Autodesk Inventor part; units mm, degrees
ref_plane "Work Plane2" through (46, 0, 0) normal (1, 0, 0) x (0, 1, 0)
ref_plane "XZ Plane" through (0, 0, 0) normal (0, 1, 0) x (-1, 0, 0)
ref_plane "XY Plane" through (0, 0, 0) normal (0, 0, 1) x (1, 0, 0)
sketch "Sketch1" plane through (0, 0, 0) normal (0, 1, 0) x (-1, 0, 0)
  circle A0 centre (0, 0) radius 46
  dimension "d0" = 92
extrude "Extrusion1" add sketch "Sketch1" along normal blind 20
sketch "Sketch2" plane through (0, 20, 0) normal (0, 1, 0) x (1, 0, 0)
  circle A0 centre (0, 0) radius 33
  dimension "d3" = 66
extrude "Extrusion2" cut sketch "Sketch2" against normal blind 14
sketch "Sketch3" plane through (0, 6, 0) normal (0, 1, 0) x (1, 0, 0)
  circle A0 centre (0, 0) radius 2.5
  dimension "d6" = 5
extrude "Extrusion3" cut sketch "Sketch3" against normal blind 6
sketch "Sketch4" plane through (0, 0, 0) normal (0, -1, 0) x (1, 0, 0)
  circle A0 centre (0, 0) radius 12
  dimension "d9" = 24
extrude "Extrusion4" add sketch "Sketch4" along normal blind 10
sketch "Sketch5" plane through (0, 0, 0) normal (0, -1, 0) x (1, 0, 0)
  circle A0 centre (0, 0) radius 2.5
  line L0 (0, 0) -> (0, -39)
  circle A1 centre (0, -39) radius 3.5
  dimension "d12" = 39
  dimension "d13" = 7
extrude "Extrusion5" cut sketch "Sketch5" against normal blind 20 contours A1
pattern_circular "Circular Pattern1" count 6 over 360 about axis through (0, 0, 0) along (0, -1, 0) of "Extrusion5"
sketch "Sketch6" plane through (0, -10, 0) normal (0, -1, 0) x (1, 0, 0)
  circle A0 centre (0, 0) radius 2.5
  circle A1 centre (0, 0) radius 7
  dimension "d19" = 14
extrude "Extrusion6" cut sketch "Sketch6" against normal blind 10 contours A0 | A1
ref_plane "Work Plane2" through (46, 0, 0) normal (1, 0, 0) x (0, 1, 0)
sketch "Sketch8" plane through (46, 0, 0) normal (1, 0, 0) x (0, 1, 0)
  point P0 (0, 0)
  point P1 (12, 0)
  point P2 (12, 0)
hole "Hole1" at (46, 12, 0) direction (-1, 0, 0) diameter 6.647 depth 22.2 tip angle 118
properties part number "valve housing"
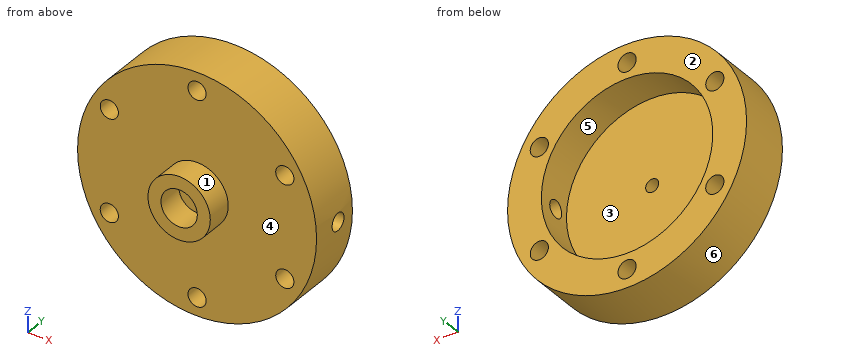
Geometry: final body of the model. Coordinates: model frame, mm. Face numbers are marked on the shaded views. A direction names the side the tool comes from. Round coordinates to 2 decimals unless told otherwise and drop trailing zeros. Loops run counter-clockwise (first coordinate to the right, second up) from the corner with the lowest first, then second, coordinate; pieces in that order, holes last. Notation, with made-up numbers: M 39,41.25 L 77,41.25 A14 cw 77,46.25 Z; hole C -18,-35 d3. An arc over 180 degrees is marked long. Put each result on its own line as item: value. Start each with the question number.
(1) Section query D-D (z = -39). Return loops of the section in (x, y).
(2) Section query C-C (y = 1.5). Return loops of the section in (x, z) (3 decimals).
(3) Material intervals for line 1 along Z through (x, y) = (0, 10.5); line 2 along X through (y, z) = (4, -19); line 3 along Y through (x, z) = (-10, -32), sorted ascending. Write a range as [from, to].
(4) Section query B-B (z = 0). Return loops of the section in (x, y), then the cut area to 3 significant figures.
(5) Contact query for flat-ended pins moving along their axis: pin 1 Ø4 at (y, z) = (12, 0) entering from +X; pin 2 Ø4 at (x, z) = (-3, 2.5) entering from -Y; pin 3 Ø10 at (x, z) = (14, 6) entering from -Y; pin 4 Ø5 at (x, y) = (-1.5, -1) entering from -Z. Output: stop coordinate, or through.
(6) Set-up query: the marked faces 4, 5 and 6. Return all of +Z, -Z, +X, -X, +Y, -Y with unobstructed straight access to the full face (end or side cutting, diameter ignored); none if empty.
(7) Draft query along Z for the marked faces 1, 2 and 3. Return one class per face: +Z half, -Z half, draft (parallel to the pull), parting line (faces both ways), or undercut.
(8) Section query A-A (x = 0). Return loops of the section in (y, z).
Findings below:
1. outline: M -24.39,0 L -3.5,0 L -3.5,20 L -24.39,20 Z; M 3.5,0 L 24.39,0 L 24.39,20 L 3.5,20 Z
2. outline: C 0,0 d92; hole C -33.775,-19.5 d7; hole C -33.775,19.5 d7; hole C 0,-39 d7; hole C 0,39 d7; hole C 0,0 d5; hole C 33.775,-19.5 d7; hole C 33.775,19.5 d7
3. line 1: z = [-46, -42.5], [-35.5, -33], [33, 35.5], [42.5, 46]
3. line 2: x = [-41.89, -37.24], [-30.31, 30.31], [37.24, 41.89]
3. line 3: y = [0, 20]
4. outline: M -46,0 L -12,0 L -12,-10 L -7,-10 L -7,0 L -2.5,0 L -2.5,6 L -33,6 L -33,20 L -46,20 Z; M 2.5,0 L 7,0 L 7,-10 L 12,-10 L 12,0 L 46,0 L 46,8.68 L 33,8.68 L 33,6 L 2.5,6 Z; M 33,15.32 L 46,15.32 L 46,20 L 33,20 Z
4. area: 900 mm2
5. pin 1: stops at x = -32.94
5. pin 2: stops at y = 0
5. pin 3: stops at y = -10
5. pin 4: stops at z = -46
6. face 4: -Y
6. face 5: +Y
6. face 6: +Y, -Y
7. face 1: parting line
7. face 2: draft
7. face 3: undercut
8. outline: M -10,-12 L 0,-12 L 0,-35.5 L 20,-35.5 L 20,-33 L 6,-33 L 6,-2.5 L 0,-2.5 L 0,-7 L -10,-7 Z; M -10,7 L 0,7 L 0,2.5 L 6,2.5 L 6,33 L 20,33 L 20,35.5 L 0,35.5 L 0,12 L -10,12 Z; M 0,-46 L 20,-46 L 20,-42.5 L 0,-42.5 Z; M 0,42.5 L 20,42.5 L 20,46 L 0,46 Z
